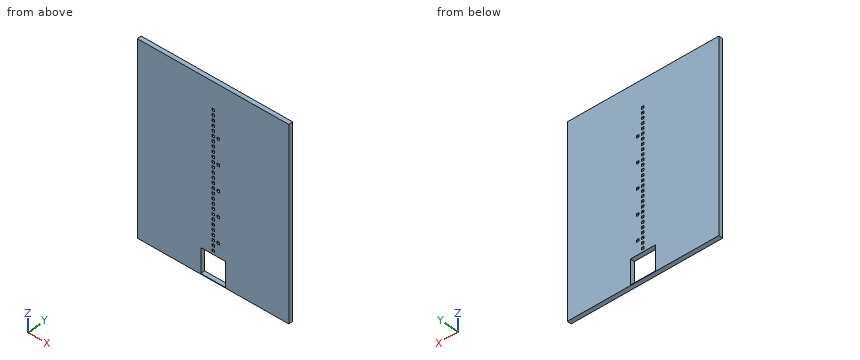
from build123d import *

# Parameters (mm, degrees)
SKETCH1_W           = 609
SKETCH1_H           = 766
SKETCH1_W_2         = 10
SKETCH1_H_2         = 10
SKETCH1_W_3         = 100
SKETCH1_H_3         = 100
BOSS_EXTRUDE1_DEPTH = 17


with BuildPart() as part:
    # Sketch1 → Boss-Extrude1 (new body)
    with BuildSketch(Plane(origin=(0, 0, 0), x_dir=(1, 0, 0), z_dir=(0, 1, 0))):
        with Locations((-0.5, -330.79)):
            Rectangle(SKETCH1_W, SKETCH1_H)
        with Locations((0, -85)):
            Rectangle(SKETCH1_W_2, SKETCH1_H_2, mode=Mode.SUBTRACT)
        Rectangle(SKETCH1_W_3, SKETCH1_H_3, mode=Mode.SUBTRACT)
        with Locations((0, -65)):
            Rectangle(SKETCH1_W_2, SKETCH1_H_2, mode=Mode.SUBTRACT)
        with Locations((0, -105)):
            Rectangle(SKETCH1_W_2, SKETCH1_H_2, mode=Mode.SUBTRACT)
        with Locations((0, -125)):
            Rectangle(SKETCH1_W_2, SKETCH1_H_2, mode=Mode.SUBTRACT)
        with Locations((0, -145)):
            Rectangle(SKETCH1_W_2, SKETCH1_H_2, mode=Mode.SUBTRACT)
        with Locations((0, -165)):
            Rectangle(SKETCH1_W_2, SKETCH1_H_2, mode=Mode.SUBTRACT)
        with Locations((0, -185)):
            Rectangle(SKETCH1_W_2, SKETCH1_H_2, mode=Mode.SUBTRACT)
        with Locations((0, -205)):
            Rectangle(SKETCH1_W_2, SKETCH1_H_2, mode=Mode.SUBTRACT)
        with Locations((0, -225)):
            Rectangle(SKETCH1_W_2, SKETCH1_H_2, mode=Mode.SUBTRACT)
        with Locations((0, -245)):
            Rectangle(SKETCH1_W_2, SKETCH1_H_2, mode=Mode.SUBTRACT)
        with Locations((0, -265)):
            Rectangle(SKETCH1_W_2, SKETCH1_H_2, mode=Mode.SUBTRACT)
        with Locations((0, -285)):
            Rectangle(SKETCH1_W_2, SKETCH1_H_2, mode=Mode.SUBTRACT)
        with Locations((0, -305)):
            Rectangle(SKETCH1_W_2, SKETCH1_H_2, mode=Mode.SUBTRACT)
        with Locations((0, -325)):
            Rectangle(SKETCH1_W_2, SKETCH1_H_2, mode=Mode.SUBTRACT)
        with Locations((0, -345)):
            Rectangle(SKETCH1_W_2, SKETCH1_H_2, mode=Mode.SUBTRACT)
        with Locations((0, -365)):
            Rectangle(SKETCH1_W_2, SKETCH1_H_2, mode=Mode.SUBTRACT)
        with Locations((0, -385)):
            Rectangle(SKETCH1_W_2, SKETCH1_H_2, mode=Mode.SUBTRACT)
        with Locations((0, -405)):
            Rectangle(SKETCH1_W_2, SKETCH1_H_2, mode=Mode.SUBTRACT)
        with Locations((0, -425)):
            Rectangle(SKETCH1_W_2, SKETCH1_H_2, mode=Mode.SUBTRACT)
        with Locations((0, -445)):
            Rectangle(SKETCH1_W_2, SKETCH1_H_2, mode=Mode.SUBTRACT)
        with Locations((0, -465)):
            Rectangle(SKETCH1_W_2, SKETCH1_H_2, mode=Mode.SUBTRACT)
        with Locations((0, -485)):
            Rectangle(SKETCH1_W_2, SKETCH1_H_2, mode=Mode.SUBTRACT)
        with Locations((0, -505)):
            Rectangle(SKETCH1_W_2, SKETCH1_H_2, mode=Mode.SUBTRACT)
        with Locations((0, -525)):
            Rectangle(SKETCH1_W_2, SKETCH1_H_2, mode=Mode.SUBTRACT)
        with Locations((0, -545)):
            Rectangle(SKETCH1_W_2, SKETCH1_H_2, mode=Mode.SUBTRACT)
        with Locations((0, -565)):
            Rectangle(SKETCH1_W_2, SKETCH1_H_2, mode=Mode.SUBTRACT)
        with Locations((0, -585)):
            Rectangle(SKETCH1_W_2, SKETCH1_H_2, mode=Mode.SUBTRACT)
        with Locations((0, -605)):
            Rectangle(SKETCH1_W_2, SKETCH1_H_2, mode=Mode.SUBTRACT)
        with Locations((20, -105)):
            Rectangle(SKETCH1_W_2, SKETCH1_H_2, mode=Mode.SUBTRACT)
        with Locations((20, -205)):
            Rectangle(SKETCH1_W_2, SKETCH1_H_2, mode=Mode.SUBTRACT)
        with Locations((20, -305)):
            Rectangle(SKETCH1_W_2, SKETCH1_H_2, mode=Mode.SUBTRACT)
        with Locations((20, -405)):
            Rectangle(SKETCH1_W_2, SKETCH1_H_2, mode=Mode.SUBTRACT)
        with Locations((20, -505)):
            Rectangle(SKETCH1_W_2, SKETCH1_H_2, mode=Mode.SUBTRACT)
    extrude(amount=BOSS_EXTRUDE1_DEPTH)


solid = part.part
Here's how the part is built. I have some questions about the finished solid (model axes, mm). Round coordinates to 2 decimals unless told otherwise and drop trailing zeros. Order: outer loops, then holes, each group sorted by start corner. A loop starts at its lowest first (then second) coordinate and runs counter-clockwise, first axis right, second up. Notation, with made-up numbers: (-12.75, 32.5) -> (38.25, 32.5) arc R19 ccw to (38.25, 37.5) -> close; hole circle Ø4 at (-29.75, 40). An arc over 180 degrees is marked (long way). Use CSV: the item, a comma, the result in double quotes.
1. I want a section at B-B on y = 7.5. Give the number of separate pieces and of enclosed holes in the cut face, and give its area (3 significant figures).
Recorded:
separate pieces,"1"
enclosed holes,"34"
area,"453,000 mm2"
2. I want a section at A-A on z = 6.5. List the corners of the cut face in (x, y) for me, and give its area (3 significant figures).
Recorded:
outline,"(-305, 0) -> (-50, 0) -> (-50, 17) -> (-305, 17) -> close; (50, 0) -> (304, 0) -> (304, 17) -> (50, 17) -> close"
area,"8,650 mm2"
3. I need wall thicknesses on line 1 along X through (y, z) = (4.75, 429); line 2 along X through (y, z) = (10.75, 41); line 3 along Z through (x, y) = (-36.5, 12.5). Which ranges of each line are inside material? Lowest first, please.
Recorded:
line 1,"x = -305 to -5, 5 to 304"
line 2,"x = -305 to -50, 50 to 304"
line 3,"z = -52.21 to -50, 50 to 713.79"
